Work out the finished part from the listing and answer in its coordinate system (mm). Give positions to 0.01 mm unless a question says otherwise; leave off trailing zeros. Loops run counter-clockwise (first coordinate to the right, second up) from the corner with the lowest first, then second, coordinate; pieces in that order, holes last.
```python
from build123d import *

# Parameters (mm, degrees)
SKETCH2_W                = 19.932631385
SKETCH2_H                = 5.9
BOSS_EXTRUDE1_DEPTH      = 4
FILLET1_R                = 1
M3_CLEARANCE_HOLE1_D     = 3.4
M3_CLEARANCE_HOLE1_DEPTH = 16.5
M3_CLEARANCE_HOLE1_TIP   = 1.021463052


with BuildPart() as part:
    # Sketch2 → Boss-Extrude1 (new body)
    with BuildSketch(Plane.XY.offset(133.365661293)):
        with Locations((-21.255805031, 37.989811256)):
            Rectangle(SKETCH2_W, SKETCH2_H)
    extrude(amount=BOSS_EXTRUDE1_DEPTH)

    # Fillet1
    fillet1_edges = [part.edges().sort_by_distance(p)[0] for p in [
        (-31.222120723, 40.939811256, 135.365661293),
        (-11.289489338, 40.939811256, 135.365661293),
        (-11.289489338, 35.039811256, 135.365661293),
        (-31.222120723, 35.039811256, 135.365661293),
    ]]
    fillet(fillet1_edges, radius=FILLET1_R)

    # M3 Clearance Hole1
    with Locations(Plane.XY.offset(137.365661293)):
        with Locations((-28.757120723, 37.989811256), (-13.757120723, 37.989811256)):
            Hole(M3_CLEARANCE_HOLE1_D / 2, depth=M3_CLEARANCE_HOLE1_DEPTH)
            with Locations((0, 0, -(M3_CLEARANCE_HOLE1_DEPTH + M3_CLEARANCE_HOLE1_TIP / 2))):  # 118° drill point
                Cone(0, M3_CLEARANCE_HOLE1_D / 2, M3_CLEARANCE_HOLE1_TIP, mode=Mode.SUBTRACT)


solid = part.part
```
Q1. Section B-B on y = 39.15 is taken. Give the vertices of the cut face in (x, z).
Q2. Consider line 1 along X through (y, z) = (37.95, 134.75); line 2 along X through (y, z) = (39.5, 136.25); line 3 along Y through (x, z) = (-13.75, 135). Determine where each line is inside the solid, lowest interval first.
Q3. Section D-D on y = 37.2 is taken. Give the vertices of the cut face in (x, z).
Q4. Determine the mould class of faces 1 (the face through (-15.38, 38.5, 135.34)), 2 (the face through (-21, 40.94, 135)), 3 (the face through (-30.937, 35.341, 135.394)) for opening direction X: +X half, -X half, draft (parallel to the pull), parting line (faces both ways), or undercut.
Q5. Section A-A on x = -29 is taken. Give the vertices of the cut face in (y, z).
Q6. Section C-C on z = 134.9 is taken. Give the vertices of the cut face in (x, y).
Check result:
1. outline: (-31.22, 133.37) - (-30, 133.37) - (-30, 137.37) - (-31.22, 137.37) - close; (-27.51, 133.37) - (-15, 133.37) - (-15, 137.37) - (-27.51, 137.37) - close; (-12.51, 133.37) - (-11.29, 133.37) - (-11.29, 137.37) - (-12.51, 137.37) - close
2. line 1: x = -31.22 to -30.46, -27.06 to -15.46, -12.06 to -11.29
2. line 2: x = -31.22 to -29.54, -27.98 to -14.54, -12.98 to -11.29
2. line 3: y = 35.04 to 36.29, 39.69 to 40.94
3. outline: (-31.22, 133.37) - (-30.26, 133.37) - (-30.26, 137.37) - (-31.22, 137.37) - close; (-27.25, 133.37) - (-15.26, 133.37) - (-15.26, 137.37) - (-27.25, 137.37) - close; (-12.25, 133.37) - (-11.29, 133.37) - (-11.29, 137.37) - (-12.25, 137.37) - close
4. face 1: undercut
4. face 2: draft
4. face 3: -X half
5. outline: (35.04, 133.37) - (36.31, 133.37) - (36.31, 137.37) - (35.04, 137.37) - close; (39.67, 133.37) - (40.94, 133.37) - (40.94, 137.37) - (39.67, 137.37) - close
6. outline: (-31.22, 36.04) arc R1 ccw to (-30.22, 35.04) - (-12.29, 35.04) arc R1 ccw to (-11.29, 36.04) - (-11.29, 39.94) arc R1 ccw to (-12.29, 40.94) - (-30.22, 40.94) arc R1 ccw to (-31.22, 39.94) - close; hole circle Ø3.4 at (-28.76, 37.99); hole circle Ø3.4 at (-13.76, 37.99)
